The listing builds one solid part. Answer for the finished solid, in the listing's coordinates (mm). A direction names the side the tool comes from. Coordinates: 2 decimals unless noted, no trailing zeros. Loops run counter-clockwise (first coordinate to the right, second up) from the corner with the lowest first, then second, coordinate; pieces in that order, holes last. Notation, with made-up numbers: (-22, -1.75) - (34, -1.75) arc R31 cw to (34, 30.25) - close; hole circle Ø1 at (16.5, 27). An arc over 180 degrees is marked (long way). Put each result on its own line as item: value.
```python
from build123d import *

# Parameters (mm, degrees)
F1_DEPTH = 12.7
F2_W     = 7.62
F2_H     = 1.3110580664
F2_H_2   = 1.3562226996
F3_DEPTH = 25.4
F4_W     = 7.62
F4_H     = 2.54
F5_DEPTH = 2.54
F7_DEPTH = 7.62


with BuildPart() as f1:
    # F0 (on Top) → F1 (new body)
    with BuildSketch(Plane.XY):
        with BuildLine():
            Line((-3.81, -0.4625546008), (-3.81, -3.175))
            Line((-3.81, -3.175), (3.81, -3.175))
            Line((3.81, -3.175), (3.81, -0.4625546008))
            Line((3.81, -0.4625546008), (3.1772142507, -0.4625546008))
            ThreePointArc((3.1772142507, -0.4625546008), (1.754829289, -0.0592090754), (3.1006408738, 0.5528838672))
            Line((3.1006408738, 0.5528838672), (3.81, 0.523305399))
            Line((3.81, 0.523305399), (3.81, 3.175))
            Line((3.81, 3.175), (-3.81, 3.175))
            Line((-3.81, 3.175), (-3.81, 0.5528838672))
            Line((-3.81, 0.5528838672), (-3.1006408738, 0.5528838672))
            ThreePointArc((-3.1006408738, 0.5528838672), (-2.2412106629, 0.7285078531), (-1.7526, 0))
            ThreePointArc((-1.7526, 0), (-2.2968372366, -0.7489129659), (-3.1772142507, -0.4625546008))
            Line((-3.1772142507, -0.4625546008), (-3.81, -0.4625546008))
        make_face()
    extrude(amount=F1_DEPTH)

    # F2 (on face) → F3 (cut)
    with BuildSketch(Plane.XY.offset(12.7)):
        with Locations((0, 2.5194709668)):
            Rectangle(F2_W, F2_H)
        with Locations((0, -2.4968886502)):
            Rectangle(F2_W, F2_H_2)
    extrude(amount=-F3_DEPTH, mode=Mode.SUBTRACT)

    # F4 (on face) → F5 (join)
    with BuildSketch(Plane.XZ.offset(1.8187773004)):
        with Locations((0, 11.43)):
            Rectangle(F4_W, F4_H)
    extrude(amount=F5_DEPTH)

    # F6 (on face) → F7 (join)
    with BuildSketch(Plane(origin=(-3.81, 0, 0), x_dir=(0, -1, 0), z_dir=(-1, 0, 0))):
        Polygon((3.0887773004, 10.16), (2.5749250781, 0), (4.3587773004, 10.16), align=None)
    extrude(amount=-F7_DEPTH)


solid = f1.part
```
1) Each of these flat-tipped pins is pushed along its axis until it touches: pin 1 (1 mm diameter, centred on x = 1.5, z = 9, fed in from -Y); pin 2 (1 mm diameter, centred on x = -1, z = 5.5, fed in from -Y); pin 3 (4 mm diameter, centred on x = 0.5, z = 4.5, fed in from -Y). Where does it stop, or does it pass through?
Found:
pin 1: stops at y = -4.24
pin 2: stops at y = -3.63
pin 3: stops at y = -3.72
2) For a pull along Z with two mould halves and no side action, classify faces 1 (the face through (3.81, 1, 6)), 2 (the face through (-0.053, -2.835, 5.151)), 3 (the face through (0, -1, 12.7)), 4 (the face through (-0.053, -3.454, 5.009)) as pulls with the +Z half, pulls with the -Z half, needs draft (parallel to the pull), parting line crosses it, or undercut.
Found:
face 1: needs draft
face 2: undercut
face 3: pulls with the +Z half
face 4: pulls with the -Z half
3) Straight lines are drawn through the part: L1, parallel to Y at x = 2.54, z = 3.25; L2, parallel to Y at x = 2, z = 2.5; L3, parallel to X at y = -0.5, z = 5.5. For each, find the intervals that lie inside material, in ascending order. Write a range as [from, to].
Found:
L1: y = [-3.15, -2.74], [-1.82, -0.79], [0.79, 1.86]
L2: y = [-3.01, -2.7], [-1.82, -0.57], [0.57, 1.86]
L3: x = [-3.81, -3.15], [-1.93, 1.93], [3.15, 3.81]
4) The part is cut by section C-C (x = 1). Give the vertices of the cut face in (y, z), and give its area (3 significant figures).
Found:
outline: (-4.36, 10.16) - (-2.57, 0) - (-3.09, 10.16) - (-1.82, 10.16) - (-1.82, 0) - (1.86, 0) - (1.86, 12.7) - (-4.36, 12.7) - close
area: 59.7 mm^2
5) The part is cut by section B-B (z = 8.5). Give the vertices of the cut face in (x, y).
Found:
outline: (-3.81, -4.07) - (3.81, -4.07) - (3.81, -3) - (-3.81, -3) - close; (-3.81, -1.82) - (3.81, -1.82) - (3.81, -0.46) - (3.18, -0.46) arc R0.79 cw (long way) to (3.1, 0.55) - (3.81, 0.52) - (3.81, 1.86) - (-3.81, 1.86) - (-3.81, 0.55) - (-3.1, 0.55) arc R0.79 cw (long way) to (-3.18, -0.46) - (-3.81, -0.46) - close
6) For faces 5 (the face through (0, -2, 10.16)), 6 (the face through (0, -1.819, 5)), 7 (the face through (-3.81, 1, 6)), determine the directions among +Z, -Z, +X, -X, +Y, -Y from which every point of the face is accessible in a straight line to the end or side of a thin tool.
Found:
face 5: +X, -X
face 6: -Z, +X, -X
face 7: +Z, -Z, -X, +Y, -Y
7) The part is cut by section A-A (x = 2.54). Give the vertices of the cut face in (y, z), and give its area (3 significant figures).
Found:
outline: (-4.36, 10.16) - (-2.57, 0) - (-3.09, 10.16) - (-1.82, 10.16) - (-1.82, 0) - (-0.79, 0) - (-0.79, 12.7) - (-4.36, 12.7) - close; (0.79, 0) - (1.86, 0) - (1.86, 12.7) - (0.79, 12.7) - close
area: 39.7 mm^2
